```python
from build123d import *

# Parameters (mm, degrees)
SKETCH1_R           = 6.5
BOSS_EXTRUDE1_DEPTH = 4
SKETCH4_R           = 2.6
CUT_EXTRUDE1_DEPTH  = 10
SKETCH5_W           = 200
SKETCH5_H           = 4
BOSS_EXTRUDE2_DEPTH = 100
FILLET1_R           = 4
SKETCH8_R           = 5
CUT_EXTRUDE2_DEPTH  = 100
SKETCH9_R           = 5
SKETCH9_R_2         = 1.75
CUT_EXTRUDE3_DEPTH  = 10
RIB1_REACH          = 249.79
SKETCH10_WALL_W     = 610.717552724
SKETCH10_WALL_H     = 4


with BuildPart() as part:
    # Sketch1 → Boss-Extrude1 (new body)
    with BuildSketch(Plane.XY):
        with BuildLine():
            Line((100, -4), (100, 0))
            Line((100, 0), (36.695562583, 145.919663525))
            ThreePointArc((36.695562583, 145.919663525), (0, 170), (-36.695562583, 145.919663525))
            Line((-36.695562583, 145.919663525), (-100, 0))
            Line((-100, 0), (-100, -4))
            Line((-100, -4), (100, -4))
        make_face()
        with Locations((0, 130)):
            Circle(SKETCH1_R, mode=Mode.SUBTRACT)
    extrude(amount=BOSS_EXTRUDE1_DEPTH)

    # Sketch4 → Cut-Extrude1 (cut)
    with BuildSketch(Plane(origin=(0, 0, 0), x_dir=(-1, 0, 0), z_dir=(0, 0, -1))):
        with Locations((0, 111.75)):
            Circle(SKETCH4_R)
        with Locations((0, 148.25)):
            Circle(SKETCH4_R)
    extrude(amount=-CUT_EXTRUDE1_DEPTH, mode=Mode.SUBTRACT)

    # Sketch5 → Boss-Extrude2 (add)
    with BuildSketch(Plane(origin=(0, 0, 0), x_dir=(-1, 0, 0), z_dir=(0, 0, -1))):
        with Locations((0, -2)):
            Rectangle(SKETCH5_W, SKETCH5_H)
    extrude(amount=-BOSS_EXTRUDE2_DEPTH)

    # Fillet1
    fillet1_edges = [part.edges().sort_by_distance(p)[0] for p in [
        (0, -4, 0),
        (0, 0, 4),
    ]]
    fillet(fillet1_edges, radius=FILLET1_R)

    # Sketch8 → Cut-Extrude2 (cut)
    with BuildSketch(Plane(origin=(0, 0, 0), x_dir=(1, 0, 0), z_dir=(0, 1, 0))):
        with Locations(Location((-85, -80, 0), (0, 0, 270))):
            Circle(SKETCH8_R)
        with Locations(Location((-85, -20, 0), (0, 0, 270))):
            Circle(SKETCH8_R)
        with Locations(Location((85, -80, 0), (0, 0, 270))):
            Circle(SKETCH8_R)
        with Locations(Location((85, -20, 0), (0, 0, 270))):
            Circle(SKETCH8_R)
    extrude(amount=-CUT_EXTRUDE2_DEPTH, mode=Mode.SUBTRACT)

    # Sketch9 → Cut-Extrude3 (cut)
    with BuildSketch(Plane.XY.offset(4)):
        with Locations((0, 25)):
            Circle(SKETCH9_R)
        with Locations((0, 33)):
            Circle(SKETCH9_R_2)
        with Locations((0, 17)):
            Circle(SKETCH9_R_2)
        with Locations((8, 25)):
            Circle(SKETCH9_R_2)
        with Locations((-8, 25)):
            Circle(SKETCH9_R_2)
    extrude(amount=-CUT_EXTRUDE3_DEPTH, mode=Mode.SUBTRACT)

    # Sketch10 wall → Rib1 (add, up to next)
    with BuildSketch(Plane(origin=(-50, 40, 40), x_dir=(0, 0.707106781187, -0.707106781187), z_dir=(0, -0.707106781187, -0.707106781187)), mode=Mode.PRIVATE) as rib1_sk1:
        Rectangle(SKETCH10_WALL_W, SKETCH10_WALL_H)
    rib1_tool1 = extrude(rib1_sk1.sketch, amount=RIB1_REACH, mode=Mode.PRIVATE) - part.part
    rib1 = rib1_tool1.solids().sort_by_distance((-50, 40, 40))[0]
    add(rib1)

    # Mirror1: Rib1 across plane
    add(rib1.mirror(Plane(origin=(0, 0, 0), x_dir=(0, 0, 1), z_dir=(1, 0, 0))))


solid = part.part
```
CAD build for the part. Positions are in the model's coordinates, mm. A direction names the side the tool comes from. Round coordinates to 2 decimals unless told otherwise and drop trailing zeros. Order: outer loops, then holes, each group sorted by start corner. A loop starts at its lowest first (then second) coordinate and runs counter-clockwise, first axis right, second up.
Item 1: Pin check, flat tips, straight feed: pin 1 (23 mm diameter, centred on y = 38.5, z = 40, fed in from -X); pin 2 (1 mm diameter, centred on x = -61, y = 78, fed in from +Z); pin 3 (13 mm diameter, centred on x = 85, z = 80, fed in from +Y). Stop position of each tip, or through.
Item 2: Saw through at D-D on x = -24. Write the cut outline in (y, z), then the cut area to 3 significant figures.
Item 3: Saw through at A-A on z = 20. Write the cut outline in (x, y).
Item 4: Tool access for faces 4 (the face through (-52, 23, 28)), 5 (the face through (48, 23, 28)), 6 (the face through (0.56, 145.71, 1.97)): list every direction of +Z, -Z, +X, -X, +Y, -Y with a clear straight run to the whole face (end or side of a thin tool).
Item 5: Mould opens along X. For faces 1 (the face through (50, 37, 43)), 2 (the face through (-86.915, -1.972, 84.619)), 3 (the face through (68.79, 71.94, 2.17)) say: pulls with the +X half, pulls with the -X half, needs draft (parallel to the pull), parting line crosses it, or undercut.
Item 6: Saw through at C-C on x = -85. Write the cut outline in (y, z).
Item 7: Probe line 1 along X through (y, z) = (-2, 80); line 2 along X through (y, z) = (32.5, 45.5); line 3 along Z through (x, y) = (35.5, 140.5). List the from-to ranges inside material, lowest first.
Item 8: Saw through at B-B on y = 111.75. Write the cut outline in (x, z).
Reported:
1. pin 1: stops at x = -52
1. pin 2: stops at z = 4
1. pin 3: stops at y = 0
2. outline: (-4, 4) arc R4 ccw to (0, 0) - (162, 0) - (162, 4) - (4, 4) arc R4 cw to (0, 8) - (0, 100) - (-4, 100) - close
2. area: 1,050 mm2
3. outline: (-100, -4) - (-90, -4) - (-90, 0) - (-100, 0) - close; (-80, -4) - (80, -4) - (80, 0) - (52, 0) - (52, 60) - (48, 60) - (48, 0) - (-48, 0) - (-48, 60) - (-52, 60) - (-52, 0) - (-80, 0) - close; (90, -4) - (100, -4) - (100, 0) - (90, 0) - close
4. face 4: +Z, -X, +Y
4. face 5: +Z, +Y
4. face 6: +Z, -Z
5. face 1: needs draft
5. face 2: undercut
5. face 3: pulls with the +X half
6. outline: (-4, 4) arc R4 ccw to (0, 0) - (34.58, 0) - (34.58, 4) - (4, 4) arc R4 cw to (0, 8) - (0, 15) - (-4, 15) - close; (-4, 25) - (0, 25) - (0, 75) - (-4, 75) - close; (-4, 85) - (0, 85) - (0, 100) - (-4, 100) - close
7. line 1: x = -100 to -90, -80 to 80, 90 to 100
7. line 2: x = -52 to -48, 48 to 52
7. line 3: z = 0 to 4
8. outline: (-51.52, 0) - (-2.6, 0) - (-2.6, 4) - (-51.52, 4) - close; (2.6, 0) - (51.52, 0) - (51.52, 4) - (2.6, 4) - close
